Study the drawing (mm; zero at the part's minimum x, y, z) and answer. A direction names the side the tool comes from. Give positions to 0.01 mm unless a question says otherwise; leave off trailing zeros. Order: outer loops, then holes, each group sorted by start corner. A loop starts at its lowest first (then second) coordinate and runs counter-clockwise, first axis right, second up.
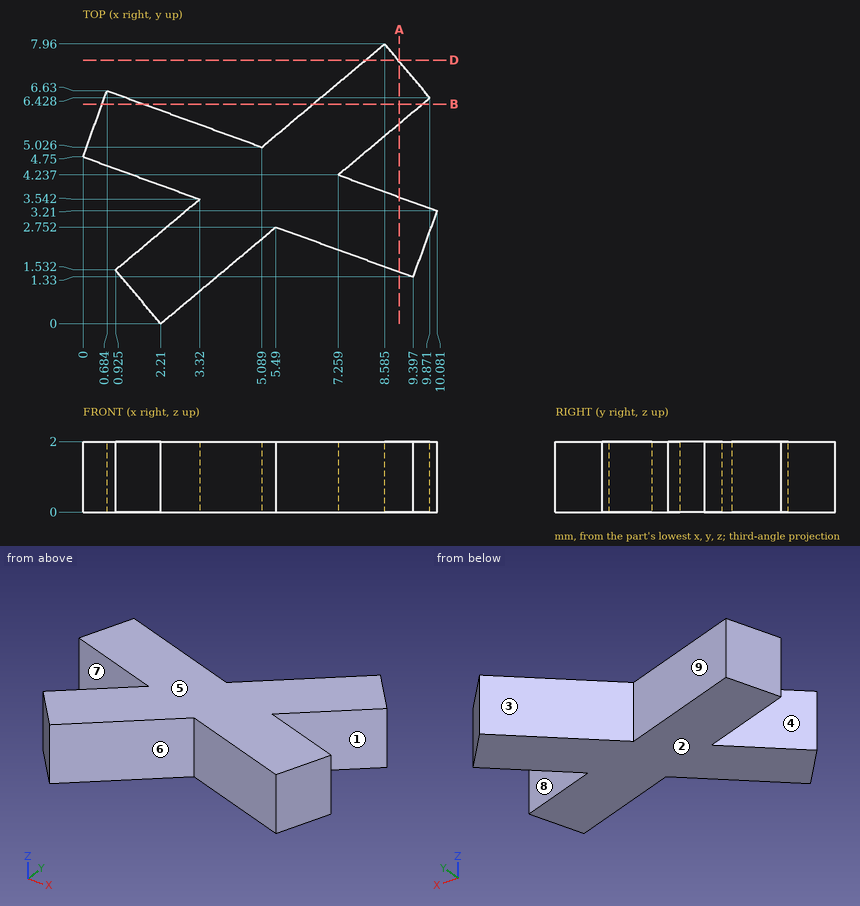
1) Straight lines are drawn through the part: probe 1 along Y at (x, z) = (9.25, 0.65) (1 decimal); probe 2 along Y at (x, z) = (3, 1.5) (1 decimal); probe 3 along X at (y, z) = (7.75, 0.5) (1 decimal). For each, find the intervals that lie inside material, in ascending order.
Geometry says:
probe 1: y = 1.4 to 3.5, 5.9 to 7.2
probe 2: y = 0.7 to 3.3, 3.7 to 5.8
probe 3: x = 8.3 to 8.8
2) Find section B-B (y = 6.25). Write down the section's boundary in (x, z) (1 decimal).
Geometry says:
outline: (0.5, 0) - (1.7, 0) - (1.7, 2) - (0.5, 2) - close; (6.5, 0) - (9.7, 0) - (9.7, 2) - (6.5, 2) - close
3) Given P1, Ø1, axis at y = 7, z = 1, coming from the +X side, flat-ended and moving along its own axis, determine where the tip first touches the part or whether it passes through.
Geometry says:
P1: stops at x = 9.81
4) A tool of negligible diameter and unlimited length cuts with its end or side. For the marked faces 5, 6, 7, 8 and 9, from which of +Z, -Z, +X, -X, +Y, -Y can it reach the whole face along a straight path? Write none if from no direction.
Geometry says:
face 5: +Z, +X, -X, +Y, -Y
face 6: +Z, -Z, -Y
face 7: +Z, -Z, -X
face 8: +Z, -Z, +X
face 9: +Z, -Z, +Y
5) Find section A-A (x = 9). Write down the section's boundary in (y, z) (1 decimal).
Geometry says:
outline: (1.5, 0) - (3.6, 0) - (3.6, 2) - (1.5, 2) - close; (5.7, 0) - (7.5, 0) - (7.5, 2) - (5.7, 2) - close
6) For a pull along Y with two mould halves and no side action, classify the marked faces 1, 2, 3 and 4 as +Y half, -Y half, draft (parallel to the pull), parting line (faces both ways), or undercut.
Geometry says:
face 1: undercut
face 2: draft
face 3: +Y half
face 4: undercut
7) Find section D-D (y = 7.5). Write down the section's boundary in (x, z).
Geometry says:
outline: (8.04, 0) - (8.97, 0) - (8.97, 2) - (8.04, 2) - close
